```python
from build123d import *

# Parameters (mm, degrees)
F0_R          = 10
F0_R_2        = 5
F1_DEPTH      = 2
F0_R_3        = 3
F2_DEPTH      = 10
F2_DEPTH_BACK = 8
F3_D          = 1.8


with BuildPart() as f1:
    # F0 (on Front) → F1 (new body)
    with BuildSketch(Plane.XZ):
        Circle(F0_R)
        Circle(F0_R_2, mode=Mode.SUBTRACT)
    extrude(amount=-F1_DEPTH)

    # F0 (on Front) → F2 (join, two sides)
    with BuildSketch(Plane.XZ) as f2_sk:
        Circle(F0_R_2)
        Circle(F0_R_3, mode=Mode.SUBTRACT)
    extrude(amount=F2_DEPTH)
    extrude(f2_sk.sketch, amount=-F2_DEPTH_BACK)

    # F3 (through all)
    with Locations(Plane.XZ):
        with Locations((0, 8), (6.928203, -4), (-6.928203, -4)):
            Hole(F3_D / 2)


solid = f1.part
```
The listing builds one solid part. Answer for the finished solid, in the listing's coordinates (mm). A direction names the side the tool comes from. Give positions to 0.01 mm unless a question says otherwise; leave off trailing zeros. Order: outer loops, then holes, each group sorted by start corner. A loop starts at its lowest first (then second) coordinate and runs counter-clockwise, first axis right, second up. Notation, with made-up numbers: (-18, -33.5) -> (10, -33.5) arc R23 cw to (10, -22.5) -> close; hole circle Ø11 at (77.25, 62.5). An arc over 180 degrees is marked (long way). One line per item, written item: value.
1) Determine the mould class of faces 4 (the cylindrical face through (-1.08, 4.96, -4.88)), 5 (the cylindrical face through (0.12, 1.01, 8.89)), 6 (the flat face through (2, 0, 5)) for opening direction X: pulls with the +X half, pulls with the -X half, needs draft (parallel to the pull), parting line crosses it, or undercut.
Reported:
face 4: parting line crosses it
face 5: undercut
face 6: needs draft
2) Flat-ended cylindrical pins translate along their axes: P1, Ø2, axis at x = -6.93, z = -4, coming from the -Y side; P2, Ø2, axis at y = -4, z = -1, coming from the -X side; P3, Ø1, axis at x = 1, y = 5.5, coming from the +Z side; P4, Ø12, axis at x = -5, z = 5, coming from the -Y side. Find the tip coordinate at first contact, or state that the pin passes through.
Reported:
P1: stops at y = 0
P2: stops at x = -5
P3: stops at z = 4.97
P4: stops at y = -10
3) Find section A-A, the plane x = 0. Determine the outline of the cut face in (y, z), plus the area to 3 significant figures.
Reported:
outline: (-10, -5) -> (0, -5) -> (0, -10) -> (2, -10) -> (2, -5) -> (8, -5) -> (8, -3) -> (-10, -3) -> close; (-10, 3) -> (8, 3) -> (8, 5) -> (2, 5) -> (2, 7.1) -> (0, 7.1) -> (0, 5) -> (-10, 5) -> close; (0, 8.9) -> (2, 8.9) -> (2, 10) -> (0, 10) -> close
area: 88.4 mm^2
4) A tool of negligible diameter and unlimited length cuts with its end or side. For faces 1 (the flat face through (2, 2, 5)), 2 (the cylindrical face through (-6.733, 1.014, -4.879)), 3 (the cylindrical face through (-1.08, -4.93, -4.88)), from which of +Z, -Z, +X, -X, +Y, -Y can it reach the whole face along a straight path? Write none if from no direction.
Reported:
face 1: +Y
face 2: +Y, -Y
face 3: -Y
5) Find section D-D, the plane x = -2.5. Determine the outline of the cut face in (y, z).
Reported:
outline: (-10, -4.33) -> (0, -4.33) -> (0, -9.68) -> (2, -9.68) -> (2, -4.33) -> (8, -4.33) -> (8, -1.66) -> (-10, -1.66) -> close; (-10, 1.66) -> (8, 1.66) -> (8, 4.33) -> (2, 4.33) -> (2, 9.68) -> (0, 9.68) -> (0, 4.33) -> (-10, 4.33) -> close
6) Find the intervals of material crossed by line 1 (Z direction, x = 0, y = 1.5); line 2 (Z direction, x = 0, y = 5); line 3 (Y direction, x = -4.5, z = 6.5), in increasing order.
Reported:
line 1: z = -10 to -3, 3 to 7.1, 8.9 to 10
line 2: z = -5 to -3, 3 to 5
line 3: y = 0 to 2
7) Find section B-B, the plane z = 8. Determine the outline of the cut face in (x, y).
Reported:
outline: (-6, 0) -> (-0.9, 0) -> (-0.9, 2) -> (-6, 2) -> close; (0.9, 0) -> (6, 0) -> (6, 2) -> (0.9, 2) -> close
8) Find section C-C, the plane z = -4. Determine the outline of the cut face in (x, y), plus the area to 3 significant figures.
Reported:
outline: (-9.17, 0) -> (-7.83, 0) -> (-7.83, 2) -> (-9.17, 2) -> close; (-6.03, 0) -> (-3, 0) -> (-3, -10) -> (3, -10) -> (3, 0) -> (6.03, 0) -> (6.03, 2) -> (3, 2) -> (3, 8) -> (-3, 8) -> (-3, 2) -> (-6.03, 2) -> close; (7.83, 0) -> (9.17, 0) -> (9.17, 2) -> (7.83, 2) -> close
area: 125 mm^2
